Verification items for the finished model (mm, model axes). Face numbers are marked on the shaded views. A direction names the side the tool comes from. Coordinates: 2 decimals unless noted, no trailing zeros. Order: outer loops, then holes, each group sorted by start corner. A loop starts at its lowest first (then second) coordinate and runs counter-clockwise, first axis right, second up. Notation, with made-up numbers: (28.25, 14.25) -> (87.25, 14.25) arc R23 ccw to (87.25, 30.25) -> close; hole circle Ø9 at (65, 72). An arc over 180 degrees is marked (long way). Write item = value, one per line. Start each with the question number.
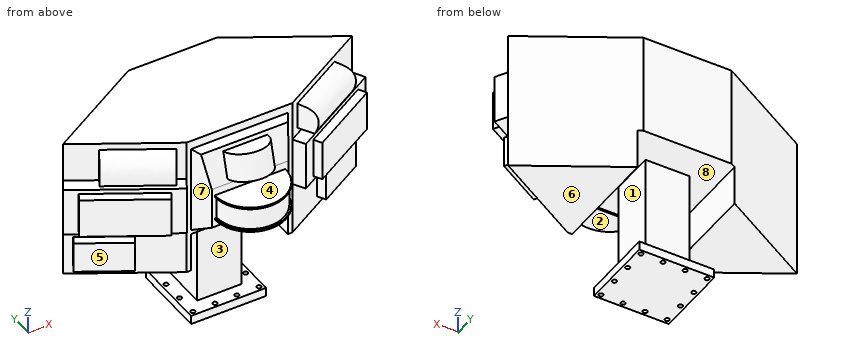
from build123d import *

# Parameters (mm, degrees)
F1_DEPTH  = 203.2
F2_W      = 76.2
F2_H      = 44.45
F3_DEPTH  = 12.7
F4_W      = 152.4
F4_H      = 69.85
F5_DEPTH  = 19.05
F6_W      = 114.3
F6_H      = 57.15
F7_DEPTH  = 12.7
F8_W      = 95.25
F8_H      = 38.1
F9_DEPTH  = 31.75
F11_DEPTH = 95.25
F12_W     = 139.7
F12_H     = 127
F13_DEPTH = 25.4
F15_DEPTH = 127
F17_DEPTH = 76.2
F19_ANGLE = 180
F20_W     = 31.75
F20_H     = 38.0410186947
F21_ANGLE = 180
F22_W     = 139.7
F22_H     = 57.15
F23_DEPTH = 159.7323484187
F25_W     = 63.5
F25_H     = 63.5
F26_DEPTH = 152.4
F27_W     = 107.95
F27_H     = 107.95
F28_DEPTH = 12.7
F29_R     = 3.175
F30_DEPTH = 12.7


with BuildPart() as f1:
    # F0 (on Top) → F1 (new body)
    with BuildSketch(Plane.XY):
        Polygon((-76.2, 0), (0, 0), (76.2, 0), (208.1822715367, 76.2), (63.5, 159.7323484187), (0, 159.7323484187), (-63.5, 159.7323484187), (-208.1822715367, 76.2), align=None)
    extrude(amount=F1_DEPTH)

    # F2 (on face) → F3 (join)
    with BuildSketch(Plane(origin=(19.05, -32.9955678842, 0), x_dir=(0.8660254038, 0.5, 0), z_dir=(0.5, -0.8660254038, 0))):
        with Locations((167.5911357684, 34.925)):
            Rectangle(F2_W, F2_H)
    extrude(amount=F3_DEPTH)

    # F4 (on face) → F5 (join)
    with BuildSketch(Plane(origin=(19.05, -32.9955678842, 0), x_dir=(0.8660254038, 0.5, 0), z_dir=(0.5, -0.8660254038, 0))):
        with Locations((142.1911357684, 111.125)):
            Rectangle(F4_W, F4_H)
    extrude(amount=F5_DEPTH)

    # F6 (on face) → F7 (join)
    with BuildSketch(Plane(origin=(28.575, -49.4933518263, 0), x_dir=(0.8660254038, 0.5, 0), z_dir=(0.5, -0.8660254038, 0))):
        with Locations((142.1911357684, 111.125)):
            Rectangle(F6_W, F6_H)
    extrude(amount=F7_DEPTH)

    # F8 (on face) → F9 (join)
    with BuildSketch(Plane(origin=(19.05, -32.9955678842, 0), x_dir=(0.8660254038, 0.5, 0), z_dir=(0.5, -0.8660254038, 0))):
        with Locations((126.3161357684, 174.625)):
            Rectangle(F8_W, F8_H)
    extrude(amount=F9_DEPTH)

    # F10 (on face) → F11 (cut, through all)
    with BuildSketch(Plane(origin=(68.1485226281, 39.3455678842, 0), x_dir=(0.5, -0.8660254038, 0), z_dir=(-0.8660254038, -0.5, 0))):
        with BuildLine():
            Line((69.85, 193.675), (38.1, 193.675))
            add(Edge.make_bspline(
                [(38.1, 193.675), (45.3948823455, 193.2153032956), (59.8621743056, 192.3554471638), (70.7391260405, 179.5930154775), (66.9907434886, 162.4530172158), (62.3683556914, 155.575)],
                knots=[0, 0, 0, 0, 0.3473900959, 0.6300376929, 1, 1, 1, 1], degree=3))
            Line((62.3683556914, 155.575), (69.85, 155.575))
            Line((69.85, 155.575), (69.85, 193.675))
        make_face()
    extrude(amount=-F11_DEPTH, mode=Mode.SUBTRACT)

    # F12 (on face) → F13 (join)
    with BuildSketch(Plane.XZ):
        with Locations((0, 127)):
            Rectangle(F12_W, F12_H)
    extrude(amount=F13_DEPTH)

    # F14 (on face) → F15 (cut, through all)
    with BuildSketch(Plane(origin=(0, 0, 63.5), x_dir=(1, 0, 0), z_dir=(0, 0, -1))):
        Polygon((69.85, 0), (69.85, 25.4), (55.1853031626, 25.4), align=None)
        Polygon((-69.85, 25.4), (-69.85, 0), (-55.1853031626, 25.4), align=None)
    extrude(amount=-F15_DEPTH, mode=Mode.SUBTRACT)

    # F16 (on Right) → F17 (cut, symmetric)
    with BuildSketch(Plane.YZ):
        Polygon((-25.4, 63.5), (0, 63.5), (-25.4, 78.1646968374), align=None)
        Polygon((-25.4, 190.5), (-25.4, 138.2009377176), (-12.2672579939, 187.2129981271), (0, 190.5), align=None)
    extrude(amount=F17_DEPTH, both=True, mode=Mode.SUBTRACT)

    # F18 (on face) → F19 (revolve)
    with BuildSketch(Plane.XZ.offset(25.4)):
        Polygon((50.8, 127.2328172775), (0, 127.2328172775), (0, 89.1328172775), (50.8, 89.1328172775), (50.8, 91.6728172775), (48.26, 91.6728172775), (48.26, 124.6928172775), (50.8, 124.6928172775), align=None)
    revolve(axis=Axis((0, -25.4, 108.1828172775), (0, 0, -1)), revolution_arc=F19_ANGLE)

    # F20 (on face) → F21 (revolve)
    with BuildSketch(Plane(origin=(0, -58.2487570575, 15.6077074137), x_dir=(1, 0, 0), z_dir=(0, -0.9659258263, 0.2588190451))):
        with Locations((15.875, 152.2883605606)):
            Rectangle(F20_W, F20_H)
    revolve(axis=Axis((0, -18.8336289969, 162.7069679224), (0, -0.2588190451, -0.9659258263)), revolution_arc=F21_ANGLE)

    # F22 (on face) → F23 (cut, through all)
    with BuildSketch(Plane.XZ):
        with Locations((0, 28.575)):
            Rectangle(F22_W, F22_H)
    extrude(amount=-F23_DEPTH, mode=Mode.SUBTRACT)

    # F24: F1 across plane


with BuildPart() as f1_1:
    add(f1.part)
    add(f1.part.mirror(Plane.YZ))

    # F25 (on face) → F26 (join)
    with BuildSketch(Plane(origin=(0, 0, 57.15), x_dir=(1, 0, 0), z_dir=(0, 0, -1))):
        with Locations((0, -79.8661742093)):
            Rectangle(F25_W, F25_H)
    extrude(amount=F26_DEPTH)

    # F27 (on face) → F28 (join)
    with BuildSketch(Plane(origin=(0, 0, -95.25), x_dir=(1, 0, 0), z_dir=(0, 0, -1))):
        with Locations((0, -79.8661742093)):
            Rectangle(F27_W, F27_H)
    extrude(amount=F28_DEPTH)

    # F29 (on face) → F30 (cut, through all)
    with BuildSketch(Plane(origin=(0, 0, -107.95), x_dir=(1, 0, 0), z_dir=(0, 0, -1))):
        with Locations((-47.625, -32.2411742093)):
            Circle(F29_R)
        with Locations((-47.625, -63.9911742093)):
            Circle(F29_R)
        with Locations((-15.875, -32.2411742093)):
            Circle(F29_R)
        with Locations((-47.625, -95.7411742093)):
            Circle(F29_R)
        with Locations((-47.625, -127.4911742093)):
            Circle(F29_R)
        with Locations((-15.875, -127.4911742093)):
            Circle(F29_R)
        with Locations((15.875, -32.2411742093)):
            Circle(F29_R)
        with Locations((47.625, -32.2411742093)):
            Circle(F29_R)
        with Locations((47.625, -63.9911742093)):
            Circle(F29_R)
        with Locations((47.625, -95.7411742093)):
            Circle(F29_R)
        with Locations((47.625, -127.4911742093)):
            Circle(F29_R)
        with Locations((15.875, -127.4911742093)):
            Circle(F29_R)
    extrude(amount=-F30_DEPTH, mode=Mode.SUBTRACT)


solid = f1_1.part
Item 1: Gauge pin test, flat ends, axial feed: P1, Ø2, axis at y = 10, z = 37, coming from the -X side; P2, Ø4, axis at x = 47.62, y = 127.49, coming from the -Z side; P3, Ø12, axis at x = -102.5, y = 38.5, coming from the -Z side. Record the tip position at first contact, or that the pin passes through.
Item 2: Tool access check on the marked faces 1, 2, 3, 4 and 5. Record the directions out of +Z, -Z, +X, -X, +Y, -Y that give a thin tool (end or side, any length) a straight path to the whole face; none if there is none.
Item 3: Section check A-A (z = 41). Record the boundary of the cut face in (x, y).
Item 4: Mould release check, pull along Z, two halves, no side actions. Record for the marked faces 6, 7 and 8: pulls with the +Z half, pulls with the -Z half, needs draft (parallel to the pull), parting line crosses it, or undercut.
Item 5: Thickness scan on line 1 (Z direction, x = 0, y = 127); line 2 (Z direction, x = -148, y = 34) (3 decimals); line 3 (X direction, y = 81, z = -50). Record the ranges inside material, lowest first.
Item 6: Section check C-C (z = -59). Record the boundary of the cut face in (x, y).
Filled sheet:
q1.P1 = -95.25
q1.P2 = 57.15
q1.P3 = 0
q2.face_1 = +Y, -Y
q2.face_2 = -Z, +X, -X, -Y
q2.face_3 = -Y
q2.face_4 = +X, -X, -Y
q2.face_5 = -Z, -X, -Y
q3.outline = (-208.18, 76.2) -> (-197.18, 69.85) -> (-203.53, 58.85) -> (-137.54, 20.75) -> (-131.19, 31.75) -> (-76.2, 0) -> (-69.85, 0) -> (-69.85, 156.07) -> close; (-31.75, 48.12) -> (31.75, 48.12) -> (31.75, 111.62) -> (-31.75, 111.62) -> close; (69.85, 0) -> (76.2, 0) -> (131.19, 31.75) -> (137.54, 20.75) -> (203.53, 58.85) -> (197.18, 69.85) -> (208.18, 76.2) -> (69.85, 156.07) -> close
q4.face_6 = pulls with the -Z half
q4.face_7 = needs draft
q4.face_8 = undercut
q5.line_1 = -107.95 to -95.25, 57.15 to 203.2
q5.line_2 = 12.7 to 57.15, 76.2 to 146.05, 155.575 to 193.218
q5.line_3 = -31.75 to 31.75
q6.outline = (-31.75, 48.12) -> (31.75, 48.12) -> (31.75, 111.62) -> (-31.75, 111.62) -> close
